```python
from build123d import *

# Parameters (mm, degrees)
SKETCH1_W           = 111
SKETCH1_H           = 85
BOSS_EXTRUDE2_DEPTH = 10
BOSS_EXTRUDE3_DEPTH = 10
SKETCH6_W           = 164
SKETCH6_H           = 158
BOSS_EXTRUDE4_DEPTH = 4
SKETCH9_R           = 2
CUT_EXTRUDE2_DEPTH  = 4
SKETCH10_W          = 186.872555015
SKETCH10_H          = 195.411118235
SKETCH10_RX         = 90
SKETCH10_RY         = 82
CUT_EXTRUDE3_DEPTH  = 4
SKETCH12_W          = 135.891970627
SKETCH12_H          = 13.567997068
CUT_EXTRUDE4_DEPTH  = 4
SKETCH13_W          = 129.508722698
SKETCH13_H          = 20.729944062
CUT_EXTRUDE5_DEPTH  = 4
SKETCH15_W          = 21.747653555
SKETCH15_H          = 111.151158821
SKETCH15_W_2        = 52.162007652
SKETCH15_H_2        = 113.873917653
CUT_EXTRUDE6_DEPTH  = 4


with BuildPart() as part:
    # Sketch1 → Boss-Extrude2 (new body)
    with BuildSketch(Plane(origin=(0, 0, 0), x_dir=(1, 0, 0), z_dir=(0, 1, 0))):
        Polygon((0, 89), (0, 0), (115, 0), (115, 89), (112, 89), (64, 89), (62, 89), align=None)
        with Locations((57.5, 44.5)):
            Rectangle(SKETCH1_W, SKETCH1_H, mode=Mode.SUBTRACT)
    extrude(amount=BOSS_EXTRUDE2_DEPTH)

    # Sketch5 → Boss-Extrude3 (add)
    with BuildSketch(Plane(origin=(0, 10, 0), x_dir=(1, 0, 0), z_dir=(0, 1, 0))):
        Polygon((54, 89), (54, 108), (0, 108), (0, 89), (2, 89), (2, 106), (52, 106), (52, 89), align=None)
    extrude(amount=-BOSS_EXTRUDE3_DEPTH)

    # Sketch6 → Boss-Extrude4 (add)
    with BuildSketch(Plane(origin=(0, 10, 0), x_dir=(1, 0, 0), z_dir=(0, 1, 0))):
        with Locations((57, 54)):
            Rectangle(SKETCH6_W, SKETCH6_H)
    extrude(amount=BOSS_EXTRUDE4_DEPTH)

    # Sketch9 → Cut-Extrude2 (cut)
    with BuildSketch(Plane.XZ.offset(-10)):
        with Locations((2, 3)):
            Circle(SKETCH9_R)
        with Locations((8.9, 3)):
            Circle(SKETCH9_R)
        with Locations((15.8, 3)):
            Circle(SKETCH9_R)
        with Locations((22.7, 3)):
            Circle(SKETCH9_R)
        with Locations((29.6, 3)):
            Circle(SKETCH9_R)
        with Locations((36.5, 3)):
            Circle(SKETCH9_R)
        with Locations((43.4, 3)):
            Circle(SKETCH9_R)
        with Locations((50.3, 3)):
            Circle(SKETCH9_R)
        with Locations((57.2, 3)):
            Circle(SKETCH9_R)
        with Locations((64.1, 3)):
            Circle(SKETCH9_R)
        with Locations((71, 3)):
            Circle(SKETCH9_R)
        with Locations((77.9, 3)):
            Circle(SKETCH9_R)
        with Locations((-3, -2)):
            Circle(SKETCH9_R)
        with Locations((-3, -10)):
            Circle(SKETCH9_R)
        with Locations((-3, -18)):
            Circle(SKETCH9_R)
        with Locations((-3, -26)):
            Circle(SKETCH9_R)
        with Locations((-3, -34)):
            Circle(SKETCH9_R)
        with Locations((-3, -42)):
            Circle(SKETCH9_R)
        with Locations((-3, -50)):
            Circle(SKETCH9_R)
        with Locations((-3, -58)):
            Circle(SKETCH9_R)
        with Locations((-3, -66)):
            Circle(SKETCH9_R)
        with Locations((-3, -74)):
            Circle(SKETCH9_R)
        with Locations((-3, -82)):
            Circle(SKETCH9_R)
        with Locations((-3, -90)):
            Circle(SKETCH9_R)
        with Locations((-3, -98)):
            Circle(SKETCH9_R)
        with Locations((-3, -106)):
            Circle(SKETCH9_R)
        with Locations((118, -2)):
            Circle(SKETCH9_R)
        with Locations((118, -9.7)):
            Circle(SKETCH9_R)
        with Locations((118, -17.4)):
            Circle(SKETCH9_R)
        with Locations((118, -25.1)):
            Circle(SKETCH9_R)
        with Locations((118, -32.8)):
            Circle(SKETCH9_R)
        with Locations((118, -40.5)):
            Circle(SKETCH9_R)
        with Locations((118, -48.2)):
            Circle(SKETCH9_R)
        with Locations((118, -55.9)):
            Circle(SKETCH9_R)
        with Locations((118, -63.6)):
            Circle(SKETCH9_R)
        with Locations((118, -71.3)):
            Circle(SKETCH9_R)
        with Locations((118, -79)):
            Circle(SKETCH9_R)
        with Locations((118, -86.7)):
            Circle(SKETCH9_R)
        with Locations((2, -111)):
            Circle(SKETCH9_R)
        with Locations((8.9, -111)):
            Circle(SKETCH9_R)
        with Locations((15.8, -111)):
            Circle(SKETCH9_R)
        with Locations((22.7, -111)):
            Circle(SKETCH9_R)
        with Locations((29.6, -111)):
            Circle(SKETCH9_R)
        with Locations((36.5, -111)):
            Circle(SKETCH9_R)
        with Locations((43.4, -111)):
            Circle(SKETCH9_R)
        with Locations((50.3, -111)):
            Circle(SKETCH9_R)
        with Locations((57, -106)):
            Circle(SKETCH9_R)
        with Locations((57, -99)):
            Circle(SKETCH9_R)
        with Locations((57, -92)):
            Circle(SKETCH9_R)
        with Locations((111.916693377, -92)):
            Circle(SKETCH9_R)
        with Locations((104.916693377, -92)):
            Circle(SKETCH9_R)
        with Locations((97.916693377, -92)):
            Circle(SKETCH9_R)
        with Locations((90.916693377, -92)):
            Circle(SKETCH9_R)
        with Locations((83.916693377, -92)):
            Circle(SKETCH9_R)
        with Locations((76.916693377, -92)):
            Circle(SKETCH9_R)
        with Locations((69.916693377, -92)):
            Circle(SKETCH9_R)
        with Locations((62.916693377, -92)):
            Circle(SKETCH9_R)
        with Locations((84.8, 3)):
            Circle(SKETCH9_R)
        with Locations((91.7, 3)):
            Circle(SKETCH9_R)
        with Locations((98.6, 3)):
            Circle(SKETCH9_R)
        with Locations((105.5, 3)):
            Circle(SKETCH9_R)
        with Locations((112.4, 3)):
            Circle(SKETCH9_R)
    extrude(amount=-CUT_EXTRUDE2_DEPTH, mode=Mode.SUBTRACT)

    # Sketch10 → Cut-Extrude3 (cut)
    with BuildSketch(Plane(origin=(0, 10, 0), x_dir=(-1, 0, 0), z_dir=(0, -1, 0))):
        with Locations((-60.171466338, 51.926348933)):
            Rectangle(SKETCH10_W, SKETCH10_H)
        with Locations(Location((-57, 54), (0, 0, -88.194857017))):
            Ellipse(SKETCH10_RX, SKETCH10_RY, mode=Mode.SUBTRACT)
    extrude(amount=-CUT_EXTRUDE3_DEPTH, mode=Mode.SUBTRACT)

    # Sketch12 → Cut-Extrude4 (cut)
    with BuildSketch(Plane.XZ.offset(-10)):
        with Locations((56.258000161, 20.433355362)):
            Rectangle(SKETCH12_W, SKETCH12_H)
    extrude(amount=-CUT_EXTRUDE4_DEPTH, mode=Mode.SUBTRACT)

    # Sketch13 → Cut-Extrude5 (cut)
    with BuildSketch(Plane(origin=(0, 10, 0), x_dir=(-1, 0, 0), z_dir=(0, -1, 0))):
        with Locations((-61.487926034, 132.323810054)):
            Rectangle(SKETCH13_W, SKETCH13_H)
    extrude(amount=-CUT_EXTRUDE5_DEPTH, mode=Mode.SUBTRACT)

    # Sketch15 → Cut-Extrude6 (cut)
    with BuildSketch(Plane(origin=(0, 10, 0), x_dir=(-1, 0, 0), z_dir=(0, -1, 0))):
        with Locations((19.765115189, 55.575579411)):
            Rectangle(SKETCH15_W, SKETCH15_H)
        with Locations((-148.394552911, 56.936958827)):
            Rectangle(SKETCH15_W_2, SKETCH15_H_2)
    extrude(amount=-CUT_EXTRUDE6_DEPTH, mode=Mode.SUBTRACT)


solid = part.part
```
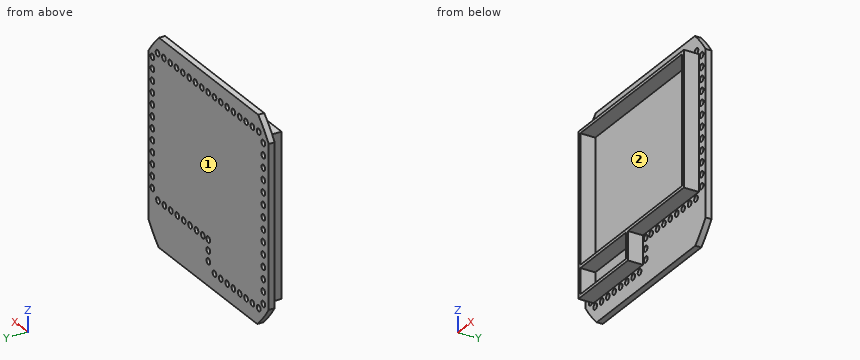
Work out the finished part from the listing and answer in its coordinate system (mm). Face numbers are marked on the shaded views. Round coordinates to 2 decimals unless told otherwise and drop trailing zeros. Write each loop counter-clockwise with the first axis right and the second up, starting at its lowest first coordinate (ties: lowest second). Pieces come first, ordered by that corner, then holes.
1) A cutting plane is placed at B-B on x = 29.6. Determine the outline of the cut face in (y, z).
2) Determine the mould class of the marked faces 1 and 2 for opening direction Z: pulls with the +Z half, pulls with the -Z half, needs draft (parallel to the pull), parting line crosses it, or undercut.
3) Flat-ended cylindrical pins translate along their axes: P1, Ø8, axis at x = 73.5, y = 7, coming from the -Z side; P2, Ø4.5, axis at x = 8.9, z = -111, coming from the -Y side; P3, Ø1, axis at x = 35.5, y = 3.5, coming from the +Z side; P4, Ø8, axis at y = 5.5, z = -98.5, coming from the +X side. Find the tip coordinate at first contact, or state that the pin passes through.
4) A cutting plane is placed at C-C on x = 57.2. Determine the outline of the cut face in (y, z).
5) A cutting plane is placed at A-A on y = 7.5. Determine the outline of the cut face in (x, z), and give its area (3 significant figures).
6) Consider probe 1 along Z at (x, y) = (46, 9.5); probe 2 along Z at (x, y) = (22.7, 11.1); probe 3 along X at (y, z) = (5, -43). Determine where each line is inside the solid, lowest interval first.
Entries:
1. outline: (0, -108) - (10, -108) - (10, -109) - (14, -109) - (14, 1) - (10, 1) - (10, 0) - (0, 0) - (0, -2) - (10, -2) - (10, -87) - (0, -87) - (0, -89) - (10, -89) - (10, -106) - (0, -106) - close; (10, -121.96) - (14, -121.96) - (14, -113) - (10, -113) - close; (10, 5) - (14, 5) - (14, 13.65) - (10, 13.65) - close
2. face 1: needs draft
2. face 2: undercut
3. P1: stops at z = -121.96
3. P2: stops at y = 10
3. P3: stops at z = 0
3. P4: stops at x = 54
4. outline: (0, -89) - (10, -89) - (10, -90.01) - (14, -90.01) - (14, 1) - (10, 1) - (10, 0) - (0, 0) - (0, -2) - (10, -2) - (10, -87) - (0, -87) - close; (10, -121.96) - (14, -121.96) - (14, -107.99) - (10, -107.99) - close; (10, -104.01) - (14, -104.01) - (14, -100.99) - (10, -100.99) - close; (10, -97.01) - (14, -97.01) - (14, -93.99) - (10, -93.99) - close; (10, 5) - (14, 5) - (14, 13.65) - (10, 13.65) - close
5. outline: (0, -108) - (54, -108) - (54, -89) - (115, -89) - (115, 0) - (0, 0) - close; hole (2, -106) - (52, -106) - (52, -89) - (2, -89) - close; hole (2, -87) - (113, -87) - (113, -2) - (2, -2) - close
5. area: 976 mm2
6. probe 1: z = -108 to -106, -89 to -87, -2 to 0
6. probe 2: z = -121.96 to -113, -109 to 1, 5 to 13.65
6. probe 3: x = 0 to 2, 113 to 115
